For this review, take the finished solid that the model builds, in its own axes (mm). Give positions to 0.01 mm unless a question says otherwise; leave off trailing zeros. Write each loop counter-clockwise with the first axis right and the second up, starting at its lowest first coordinate (ties: lowest second). Pieces come first, ordered by that corner, then holes. Notation, with made-up numbers: M -13,-2.5 L 16,-2.5 A4 cw 16,1.5 Z; hole C -3.5,-35 d9. An arc over 180 degrees is marked long. One line per item, written item: value. Start each with the question number.
Item 1: To check wall thickness, follow probe 1 along Y at (x, z) = (0, -134); probe 2 along Z at (x, y) = (4, -5); probe 3 along Z at (x, y) = (9.25, 3). State the ranges of each line that lie inside material, in increasing order.
Item 2: Clearance check with flat-ended pins moving along their axes: pin 1 Ø5 at (x, y) = (-10, 11) entering from -Z; pin 2 Ø6.5 at (y, z) = (-1, 17) entering from +X; pin 3 Ø8 at (x, z) = (-4.5, -183) entering from -Y. State where each tip first meets the part, or that it passes through.
Item 3: Consider section B-B, the plane z = -186. Write out the cut boundary in (x, y) (1 decimal).
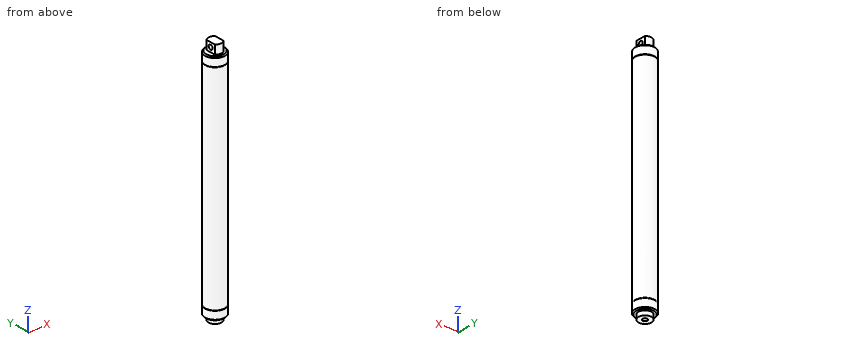
Autodesk Inventor part; units mm, degrees
ref_plane "YZ Plane" through (0, 0, 0) normal (1, 0, 0) x (0, 1, 0)
ref_plane "XZ Plane" through (0, 0, 0) normal (0, 1, 0) x (-1, 0, 0)
ref_plane "XY Plane" through (0, 0, 0) normal (0, 0, 1) x (1, 0, 0)
sketch "Sketch1" plane through (0, 0, 0) normal (0, 0, 1) x (1, 0, 0)
  circle A0 centre (0, 0) radius 12.7
  circle A1 centre (0, 0) radius 14.2875
  line L0 (-6.35, 7.0995) -> (6.35, 7.0995)
  line L1 (6.35, 7.0995) -> (6.35, -7.0995)
  line L2 (6.35, -7.0995) -> (-6.35, -7.0995)
  line L3 (-6.35, -7.0995) -> (-6.35, 7.0995)
  arc A2 (6.35, 7.0995) -> (-6.35, 7.0995) centre (0, 0) ccw
  arc A3 (-6.35, -7.0995) -> (6.35, -7.0995) centre (0, 0) ccw
  dimension "d2" = 25.4
  dimension "d3" = 28.575
  dimension "d4" = 12.7
  dimension "d5" = 6.35
  dimension "d6" = 14.199
  dimension "d7" = 7.0995
  dimension "d8" = 9.525
extrude "Extrusion1" add sketch "Sketch1" against normal blind 304.8 contours A1
fillet "Fillet1" radius 0.7937 2 edges at (-14.2875, 0, 0) (-14.2875, 0, -304.8)
extrude "Extrusion2" add sketch "Sketch1" along normal blind 12.7 contours A0 | A1
extrude "Extrusion3" add sketch "Sketch1" along normal blind 25.4 contours A2 L0 | L0 L1 L2 L3 | L2 A3
chamfer "Chamfer1" distance 1.5875 angle 45 1 edges at (-14.2875, 0, 12.7)
thread "Thread1"
thread "Thread2"
sketch "Sketch2" plane through (0, 0, -304.8) normal (0, 0, -1) x (-1, 0, 0)
  circle A0 centre (0, 0) radius 14.2875
  circle A1 centre (0, 0) radius 9.525
  circle A2 centre (0, 0) radius 3.175
  circle A3 centre (0, 0) radius 3.9688
  dimension "d24" = 19.05
  dimension "d25" = 7.9375
  dimension "d26" = 6.35
extrude "Extrusion4" add sketch "Sketch2" along normal blind 12.7 contours A0
extrude "Extrusion5" add sketch "Sketch2" along normal blind 19.05 contours A3
fillet "Fillet2" radius 0.1905 2 edges at (3.9688, 0, -323.85) (3.175, 0, -323.85)
extrude "Extrusion6" add sketch "Sketch2" along normal blind 19.05 contours A1
chamfer "Chamfer2" distance 1.5875 angle 45 1 edges at (14.2875, 0, -317.5)
thread "Thread3"
sketch "Sketch3" plane through (6.35, -7.0995, 12.7) normal (1, 0, 0) x (0, 0, -1)
  line L0 (0, 14.199) -> (-12.7, 14.199)
  line L1 (-12.7, 14.199) -> (-12.7, 0)
  line L2 (0, 0) -> (-12.7, 0)
  circle A0 centre (-6.35, 7.0995) radius 3.175
  point P0 (12.7, 7.0995)
  dimension "d39" = 6.35
  dimension "d40" = 7.0995
  dimension "d41" = 14.199
  dimension "d42" = 6.35
extrude "Extrusion7" cut sketch "Sketch3" against normal blind 25.4
equation "\"d40\" = 0.5 * d41"
properties part number "1' by 1'' dia piston"
Model answer:
1. probe 1: y = -14.29 to -12.7, 12.7 to 14.29
1. probe 2: z = -323.85 to -304.8, 0 to 25.4
1. probe 3: z = -317.5 to -304.8, 0 to 12.7
2. pin 1: stops at z = -317.5
2. pin 2: stops at x = 6.35
2. pin 3: stops at y = -14.28
3. outline: C 0,0 d28.6; hole C 0,0 d25.4
